from build123d import *

# Parameters (mm, degrees)
F1_DEPTH = 31.75
F3_R     = 1.27


# Not quite as in the source:
# - a feature names something its author has since deleted; it is built from what else it names


with BuildPart() as f1:
    # F0 (on Front) → F1 (new body)
    with BuildSketch(Plane.XZ):
        Polygon((3.556, 2.0828), (-3.556, 2.0828), (-3.556, 0), (-7.4295, 0), (-7.4295, -2.032), (-2.54, -5.334), (2.54, -5.334), (7.4295, -2.032), (7.4295, 0), (3.556, 0), align=None)
    extrude(amount=F1_DEPTH)

    # F3
    f3_edges = [f1.edges().sort_by_distance(p)[0] for p in [
        (7.4295, -15.875, -2.032),
        (2.54, -15.875, -5.334),
        (-2.54, -15.875, -5.334),
        (-7.4295, -15.875, -2.032),
    ]]
    fillet(f3_edges, radius=F3_R)


solid = f1.part
Design review of the part built by this model. Coordinates are the model's own, in mm. A direction names the side the tool comes from. Coordinates: 2 decimals unless noted, no trailing zeros. Loops run counter-clockwise (first coordinate to the right, second up) from the corner with the lowest first, then second, coordinate; pieces in that order, holes last.
Item 1: Add section B-B (x = 6.5). Write out the cut boundary in (y, z).
Completed:
outline: (-31.75, -2.66) - (0, -2.66) - (0, 0) - (-31.75, 0) - close
Item 2: Add section C-C (z = -3.25). Write out the cut boundary in (x, y).
Completed:
outline: (-5.63, -31.75) - (5.63, -31.75) - (5.63, 0) - (-5.63, 0) - close
Item 3: Add section A-A (y = -30). Write out the cut boundary in (x, z).
Completed:
outline: (-7.43, -1.36) arc R1.27 ccw to (-6.87, -2.41) - (-2.86, -5.12) arc R1.27 ccw to (-2.15, -5.33) - (2.15, -5.33) arc R1.27 ccw to (2.86, -5.12) - (6.87, -2.41) arc R1.27 ccw to (7.43, -1.36) - (7.43, 0) - (3.56, 0) - (3.56, 2.08) - (-3.56, 2.08) - (-3.56, 0) - (-7.43, 0) - close
Item 4: For faces 1 (the flat face through (-3.556, -16, 1)), 2 (the flat face through (0, -31.75, -2)), 3 (the flat face through (3.556, -16, 1)), list the 3-axis set-ups (+Z, -Z, +X, -X, +Y, -Y) from which the entire face can be reached by the end or side of a thin tool; tool diameter is ignored.
Completed:
face 1: +Z, -X, +Y, -Y
face 2: +Z, -Z, +X, -X, -Y
face 3: +Z, +X, +Y, -Y
Item 5: Wall thickness on L1, parallel to X at y = -17, z = 0.75; L2, parallel to X at y = -13.5, z = -2.5; L3, parallel to Z at x = 4.25, y = -21: over which ranges is each line inside the solid? List them lowest first.
Completed:
L1: x = -3.56 to 3.56
L2: x = -6.74 to 6.74
L3: z = -4.18 to 0
Item 6: Clearance check with flat-ended pins moving along their axes: pin 1 (1.9 mm diameter, centred on x = -6.5, y = -14, fed in from +Z); pin 2 (1 mm diameter, centred on y = -19, z = 1, fed in from +X). State where each tip first meets the part, or that it passes through.
Completed:
pin 1: stops at z = 0
pin 2: stops at x = 3.56
